Could you check a few things on this model? Use its own coordinates, in mm. A direction names the side the tool comes from. Coordinates: 2 decimals unless noted, no trailing zeros. Loops run counter-clockwise (first coordinate to the right, second up) from the corner with the lowest first, then second, coordinate; pieces in that order, holes last. Notation, with made-up numbers: (31.25, 38) - (68.25, 38) arc R22 cw to (68.25, 44) - close; hole circle Ø11 at (76, -3.5). An arc over 180 degrees is marked (long way). One line per question, with ' | ' between items. Start each with the question number.
1. Which directions (+Z, -Z, +X, -X, +Y, -Y) give clear straight access to the entire face, cutting with the end or side of a thin tool? Please do faces 1 (the flat face through (-49.32, 82.6, 120.03)), 2 (the flat face through (-2, 300, 2)), 3 (the flat face through (80, 5, -104)).
2. We'd pull the mould along Z, two halves only. Please class faces 4 (the flat face through (-120.03, 83.51, 49.32)), 5 (the cylindrical face through (-0.98, 2.54, 149.39)), 6 (the cylindrical face through (124.95, 157.1, -39.35)), 7 (the flat face through (116, 0, -57)): pulls with the +Z half, pulls with the -Z half, needs draft (parallel to the pull), parting line crosses it, or undercut.
3. I want a section at D-D, the plane y = 219.5. Write out the boundary of the cut face in (x, z).
4. I'm going to push flat-ended pins straight in: P1, Ø4, axis at x = 102, y = 226.5, coming from the -Z side; P2, Ø3, axis at x = -42, y = 211.5, coming from the +Z side; P3, Ø10, axis at x = -82, y = 165, coming from the +Z side; P4, Ø7, axis at x = -145, z = 0, coming from the -Y side. Where does each tip first touch, or does it pass through?
5. I want a section at C-C, the plane z = -145. Write out the boundary of the cut face in (x, y), then the cut area to 3 significant figures.
6. I want a section at B-B, the plane z = 0. Write out the boundary of the cut face in (x, y).
7. Please list where these lines run through material, in increasing order: L1, parallel to X at y = 1.8, z = 0; L2, parallel to Z at x = 0, y = 162. Write a range as [from, to].
8. I want a section at A-A, the plane x = 0. Write out the boundary of the cut face in (y, z).
Autodesk Inventor part; units mm, degrees
ref_plane "Work Plane2" through (-109.6016, 0, 109.6016) normal (0.7071, 0, -0.7071) x (0, 1, 0)
ref_plane "XZ Plane" through (0, 0, 0) normal (0, 1, 0) x (-1, 0, 0)
ref_plane "XY Plane" through (0, 0, 0) normal (0, 0, 1) x (1, 0, 0)
sketch "Sketch1" plane through (0, 0, 0) normal (0, 1, 0) x (-1, 0, 0)
  circle A0 centre (0, 0) radius 155
  dimension "d0" = 310
extrude "Extrusion1" add sketch "Sketch1" along normal blind 305
sketch "Sketch2" plane through (0, 305, 0) normal (0, 1, 0) x (1, 0, 0)
  circle A0 centre (0, 0) radius 131
  circle A1 centre (0, 0) radius 155
  dimension "d3" = 262
  dimension "d4" = 310
extrude "Extrusion2" cut sketch "Sketch2" against normal blind 300
sketch "Sketch3" plane through (0, 0, 0) normal (0, -1, 0) x (1, 0, 0)
  circle A0 centre (0, 0) radius 126
  dimension "d7" = 252
extrude "Extrusion3" cut sketch "Sketch3" against normal blind 300
sketch "Sketch4" plane through (0, 5, 0) normal (0, 1, 0) x (1, 0, 0)
  circle A0 centre (0, 0) radius 155
  line L0 (-155, 0) -> (-145, 0)
  line L1 (-155, 0) -> (-145, 0) construction
  circle A1 centre (-145, 0) radius 4.5
  circle A2 centre (0, -145) radius 4.5
  line L2 (0, -155) -> (0, -145)
  circle A3 centre (145, 0) radius 4.5
  line L3 (155, 0) -> (145, 0)
  circle A4 centre (0, 145) radius 4.5
  line L4 (0, 155) -> (0, 145)
  dimension "d10" = 10
  dimension "d12" = 9
  dimension "d15" = 360
extrude "Extrusion4" cut sketch "Sketch4" against normal through all contours A4 | A1 | A2 | A3
ref_plane "Work Plane2" through (-109.6016, 0, 109.6016) normal (0.7071, 0, -0.7071) x (0, 1, 0)
ref_plane "Work Plane1" through (0, 0, 0) normal (0.7071, 0, -0.7071) x (0, 1, 0)
sketch "Sketch5" plane through (-109.6016, 0, 109.6016) normal (0.7071, 0, -0.7071) x (0, 1, 0)
  line L0 (195, -50) -> (0, -50)
  line L1 (0, -50) -> (0, 50)
  line L2 (0, 50) -> (195, 50)
  line L3 (195, 50) -> (195, -50)
  line L4 (0, 155) -> (0, -155)
  point P0 (0, 0)
  dimension "d20" = 195
  dimension "d21" = 100
  dimension "d22" = 0
  dimension "d23" = 50
extrude "Extrusion5" cut sketch "Sketch5" along normal up to surface
properties part number "external_cover"
Results are:
1) face 1: -X, -Y | face 2: -Y | face 3: +Y
2) face 4: pulls with the +Z half | face 5: undercut | face 6: parting line crosses it | face 7: needs draft
3) outline: circle Ø262 at (0, 0); hole circle Ø252 at (0, 0)
4) P1: stops at z = -84.62 | P2: stops at z = 124.58 | P3: stops at z = -91.14 | P4: passes through
5) outline: (-54.77, 0) - (-4.5, 0) - (-4.5, 5) - (-54.77, 5) - close; (4.5, 0) - (54.77, 0) - (54.77, 5) - (4.5, 5) - close | area: 503 mm2
6) outline: (-155, 0) - (-149.5, 0) - (-149.5, 5) - (-155, 5) - close; (-140.5, 0) - (-126, 0) - (-126, 300) - (126, 300) - (126, 0) - (140.5, 0) - (140.5, 5) - (131, 5) - (131, 305) - (-131, 305) - (-131, 5) - (-140.5, 5) - close; (149.5, 0) - (155, 0) - (155, 5) - (149.5, 5) - close
7) L1: x = [-155, -149.5], [-140.5, -126], [126, 140.5], [149.5, 155] | L2: z = [-131, -126], [126, 131]
8) outline: (0, -155) - (5, -155) - (5, -149.5) - (0, -149.5) - close; (0, -140.5) - (5, -140.5) - (5, -131) - (305, -131) - (305, 131) - (5, 131) - (5, 140.5) - (0, 140.5) - (0, 126) - (300, 126) - (300, -126) - (0, -126) - close; (0, 149.5) - (5, 149.5) - (5, 155) - (0, 155) - close
